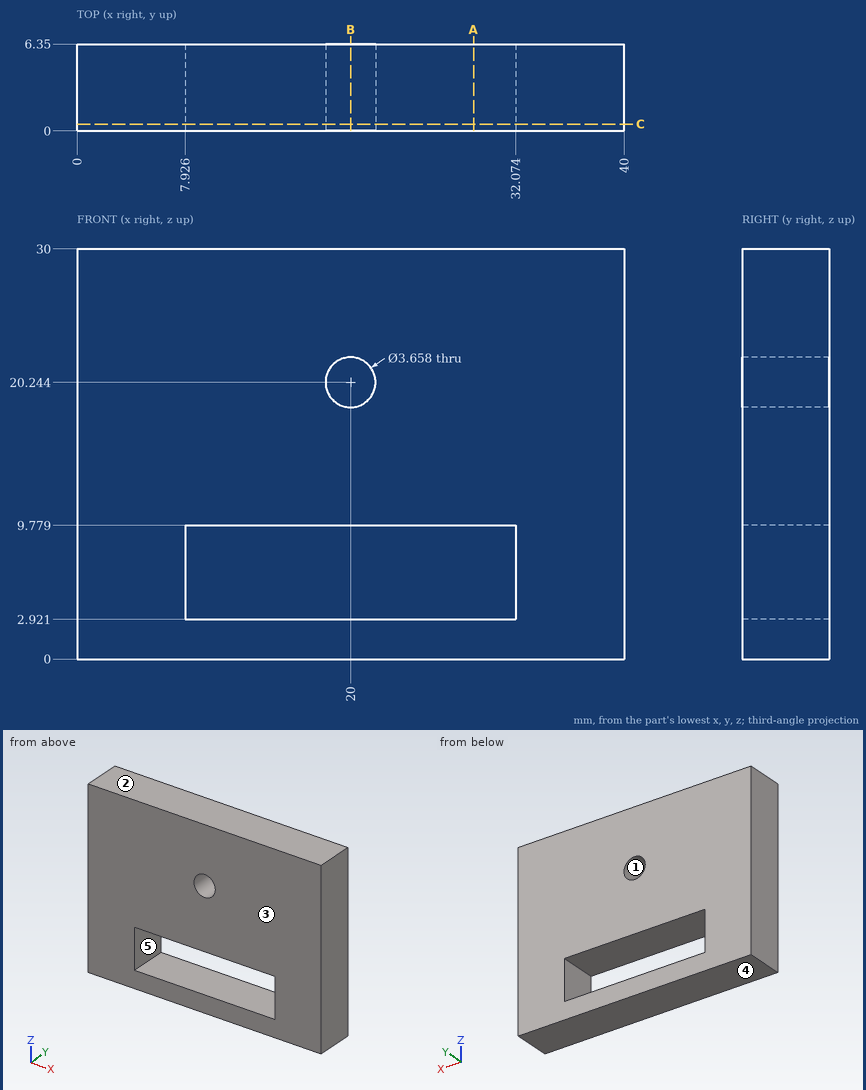
Drawing for the job (mm, zero at the part's lowest x, y, z). A direction names the side the tool comes from. Round coordinates to 2 decimals unless told otherwise and drop trailing zeros. Loops run counter-clockwise (first coordinate to the right, second up) from the corner with the lowest first, then second, coordinate; pieces in that order, holes last. Notation, with made-up numbers: (-27.75, 17.25) - (21.25, 17.25) arc R8 ccw to (21.25, 24.25) - close; hole circle Ø9 at (49, 1). An arc over 180 degrees is marked (long way). Return JSON: item names as keys, results as strings. Group by question number.
Q1. Band-saw the part on C-C on y = 0.5. Give the cut face in (x, z).
Q2. Drill centre lines: line 1 along Z through (x, y) = (20, 4) (1 decimal); line 2 along X through (y, z) = (1.5, 3.5); line 3 along Z through (x, y) = (27, 4.75). Where is each one in solid material? Low to high. Write a range as [from, to].
Q3. Tool access for the marked faces 4 and 5: list every direction of +Z, -Z, +X, -X, +Y, -Y with a clear straight run to the whole face (end or side of a thin tool).
Q4. Two-plate mould, pull along Z, no slides. Class the marked faces 1, 2 and 3: +Z half, -Z half, draft (parallel to the pull), parting line (faces both ways), or undercut.
Q5. Band-saw the part on B-B on x = 20. Give the number of separate pieces and of enclosed holes in the cut face, plus the area to 3 significant figures.
Q6. Band-saw the part on A-A on x = 29. Give the cut face in (y, z), plus the area to 3 significant figures.
Solutions:
{
 "1": {"outline": "(0, 0) - (40, 0) - (40, 30) - (0, 30) - close; hole (7.93, 2.92) - (32.07, 2.92) - (32.07, 9.78) - (7.93, 9.78) - close; hole circle Ø3.66 at (20, 20.24)"},
 "2": {"line 1": "z = [0, 2.9], [9.8, 18.4], [22.1, 30]", "line 2": "x = [0, 7.93], [32.07, 40]", "line 3": "z = [0, 2.92], [9.78, 30]"},
 "3": {"face 4": "-Z, +X, -X, +Y, -Y", "face 5": "+Y, -Y"},
 "4": {"face 1": "undercut", "face 2": "+Z half", "face 3": "draft"},
 "5": {"separate pieces": "3", "enclosed holes": "0", "area": "124 mm^2"},
 "6": {"outline": "(0, 0) - (6.35, 0) - (6.35, 2.92) - (0, 2.92) - close; (0, 9.78) - (6.35, 9.78) - (6.35, 30) - (0, 30) - close", "area": "147 mm^2"}
}
